Design review of the part built by this model. Coordinates are the model's own, in mm. A direction names the side the tool comes from. Give positions to 0.01 mm unless a question says otherwise; leave off trailing zeros. Write each loop counter-clockwise with the first axis right and the second up, starting at its lowest first coordinate (ties: lowest second). Pieces come first, ordered by that corner, then holes. Notation, with made-up numbers: M -36,18 L -14,18 A31 cw -14,53 Z; hole C -31.75,26 d11. An arc over 180 degrees is marked long. Answer in a Markdown table with one row per item.
```python
from build123d import *

# Parameters (mm, degrees)
SKETCH1_W            = 211.1756
SKETCH1_H            = 127
BOSS_EXTRUDE1_DEPTH  = 6.35
M3_CLEARANCE_HOLE1_D = 3.4
SKETCH4_W            = 3.5052
SKETCH4_H            = 47.625
CUT_EXTRUDE1_DEPTH   = 247.50447569
CUT_EXTRUDE2_DEPTH   = 247.50447569


with BuildPart() as part:
    # Sketch1 → Boss-Extrude1 (new body)
    with BuildSketch(Plane.XY):
        with Locations((105.5878, 63.5)):
            Rectangle(SKETCH1_W, SKETCH1_H)
    extrude(amount=BOSS_EXTRUDE1_DEPTH)

    # M3 Clearance Hole1 (through all)
    with Locations(Plane.XY.offset(6.35)):
        with Locations((5.9944, 105.0036), (5.9944, 66.9036), (205.1812, 66.9036), (205.1812, 105.0036)):
            Hole(M3_CLEARANCE_HOLE1_D / 2)

    # Sketch4 → Cut-Extrude1 (cut, through all)
    with BuildSketch(Plane.XY.offset(6.35)):
        with Locations((48.7426, 84.1375)):
            Rectangle(SKETCH4_W, SKETCH4_H)
        with Locations((162.433, 84.1375)):
            Rectangle(SKETCH4_W, SKETCH4_H)
    extrude(amount=-CUT_EXTRUDE1_DEPTH, mode=Mode.SUBTRACT)

    # Sketch5 → Cut-Extrude2 (cut, through all)
    with BuildSketch(Plane.XY.offset(6.35)):
        Polygon((0, 50.708311795), (89.7128, 38.1), (121.4628, 38.1), (211.1756, 50.708311795), (211.1756, 0), (0, 0), align=None)
    extrude(amount=-CUT_EXTRUDE2_DEPTH, mode=Mode.SUBTRACT)


solid = part.part
```
1) Add section C-C (x = 172.5). Write out the cut boundary in (y, z).
Geometry says:
| item | result |
|---|---|
| outline | M 45.27,0 L 127,0 L 127,6.35 L 45.27,6.35 Z |
2) Add section B-B (z = 4.75). Write out the cut boundary in (x, y) (3 decimals), and give its area (3 significant figures).
Geometry says:
| item | result |
|---|---|
| outline | M 0,50.708 L 89.713,38.1 L 121.463,38.1 L 211.176,50.708 L 211.176,127 L 0,127 Z; hole C 5.994,66.904 d3.4; hole C 5.994,105.004 d3.4; hole M 46.99,60.325 L 50.495,60.325 L 50.495,107.95 L 46.99,107.95 Z; hole M 160.68,60.325 L 164.186,60.325 L 164.186,107.95 L 160.68,107.95 Z; hole C 205.181,66.904 d3.4; hole C 205.181,105.004 d3.4 |
| area | 17,300 mm^2 |
3) Insertion check: P1, Ø3, axis at x = 162.5, z = 4.5, coming from the -Y side; P2, Ø2, axis at x = 5.99, y = 105, coming from the +Z side; P3, Ø4.5, axis at x = 205.18, y = 66.9, coming from the -Z side; P4, Ø1.5, axis at x = 40, z = 1, coming from the -Y side. Each pin has a flat end and moves straight along its axis. Give the tip position at first contact, or say it passes through.
Geometry says:
| item | result |
|---|---|
| P1 | y = 43.66 |
| P2 | through |
| P3 | z = 0 |
| P4 | y = 44.98 |
4) The part is to be moulded in two halves that separate along X. For faces 3 (the face through (0, 88, 3)), 4 (the face through (49, 107.95, 3)), 5 (the face through (46.99, 84, 3)), 6 (the face through (165.691, 44.316, 3.219)), say which applies: released by +X, released by -X, zero draft, split by the parting line, or undercut.
Geometry says:
| item | result |
|---|---|
| face 3 | released by -X |
| face 4 | undercut |
| face 5 | undercut |
| face 6 | released by +X |
5) To check wall thickness, follow probe 1 along X at (y, z) = (100.5, 4); probe 2 along X at (y, z) = (65.5, 6.25); probe 3 along X at (y, z) = (68, 5.25). State the ranges of each line that lie inside material, in increasing order. Write a range as [from, to].
Geometry says:
| item | result |
|---|---|
| probe 1 | [0, 46.99], [50.5, 160.68], [164.19, 211.18] |
| probe 2 | [0, 5.04], [6.95, 46.99], [50.5, 160.68], [164.19, 204.22], [206.14, 211.18] |
| probe 3 | [0, 4.7], [7.29, 46.99], [50.5, 160.68], [164.19, 203.88], [206.48, 211.18] |
6) Add section D-D (x = 75). Write out the cut boundary in (y, z).
Geometry says:
| item | result |
|---|---|
| outline | M 40.17,0 L 127,0 L 127,6.35 L 40.17,6.35 Z |
7) For faces 1 (the face through (164.186, 84, 3)), 2 (the face through (105, 38.1, 3)), list the 3-axis set-ups (+Z, -Z, +X, -X, +Y, -Y) from which the entire face can be reached by the end or side of a thin tool; tool diameter is ignored.
Geometry says:
| item | result |
|---|---|
| face 1 | +Z, -Z |
| face 2 | +Z, -Z, +X, -X, -Y |
8) Add section A-A (y = 73). Write out the cut boundary in (x, z), and give its area (3 significant figures).
Geometry says:
| item | result |
|---|---|
| outline | M 0,0 L 46.99,0 L 46.99,6.35 L 0,6.35 Z; M 50.5,0 L 160.68,0 L 160.68,6.35 L 50.5,6.35 Z; M 164.19,0 L 211.18,0 L 211.18,6.35 L 164.19,6.35 Z |
| area | 1,300 mm^2 |
